from build123d import *

# Parameters (mm, degrees)
SKETCH_1_W          = 54.45
SKETCH_1_H          = 10.46
SKETCH_1_H_2        = 107.75
EXTRUDE_1_DEPTH     = 24.02
CUT_EXTRUDE_1_DEPTH = 10
EXTRUDE_2_DEPTH     = 4.21
SKETCH_4_W          = 3.45
SKETCH_4_H          = 10.08
CUT_EXTRUDE_2_DEPTH = 2
SKETCH_5_W          = 6.71
SKETCH_5_H          = 4.88
CUT_EXTRUDE_4_DEPTH = 134.379468529
SKETCH_7_W          = 5.3
SKETCH_7_H          = 23.4
CUT_EXTRUDE_5_DEPTH = 0.2
SKETCH_8_W          = 10.6
SKETCH_8_H          = 9.42
CUT_EXTRUDE_6_DEPTH = 0.2
SKETCH_9_W          = 10.6
SKETCH_9_H          = 8
CUT_EXTRUDE_7_DEPTH = 0.2
SKETCH_10_W         = 6.68
SKETCH_10_H         = 5.61
CUT_EXTRUDE_8_DEPTH = 2.08


with BuildPart() as part:
    # 草图1 → 凸台-拉伸1 (new body)
    with BuildSketch(Plane(origin=(0, 0, 0), x_dir=(0, 0, -1), z_dir=(1, 0, 0))):
        with Locations((0, 53.875)):
            Rectangle(SKETCH_1_W, SKETCH_1_H)
        with Locations((0, -5.23)):
            Rectangle(SKETCH_1_W, SKETCH_1_H_2)
        Polygon((-37.585, -66.595), (27.225, -59.105), (-27.225, -59.105), (-27.225, 48.645), (-37.585, 48.645), align=None)
        Polygon((-27.225, 59.105), (-37.585, 48.645), (-27.225, 48.645), align=None)
    extrude(amount=EXTRUDE_1_DEPTH)

    # 草图2 → 切除-拉伸1 (cut)
    with BuildSketch(Plane(origin=(0, 59.105, 0), x_dir=(1, 0, 0), z_dir=(0, 1, 0))):
        with BuildLine():
            ThreePointArc((16.585, 17.36), (15.245013524, 20.595013524), (12.01, 21.935))
            Line((12.01, 21.935), (12.01, 12.785))
            ThreePointArc((12.01, 12.785), (15.245013524, 14.124986476), (16.585, 17.36))
        make_face()
        with BuildLine():
            Line((12.01, 12.785), (12.01, 21.935))
            ThreePointArc((12.01, 21.935), (7.435, 17.36), (12.01, 12.785))
        make_face()
    extrude(amount=-CUT_EXTRUDE_1_DEPTH, mode=Mode.SUBTRACT)

    # 草图3 → 凸台-拉伸2 (add)
    with BuildSketch(Plane(origin=(0, 59.105, 0), x_dir=(1, 0, 0), z_dir=(0, 1, 0))):
        with BuildLine():
            ThreePointArc((14.035, 7.04), (13.441891232, 8.471891232), (12.01, 9.065))
            Line((12.01, 9.065), (12.01, 5.015))
            ThreePointArc((12.01, 5.015), (13.441891232, 5.608108768), (14.035, 7.04))
        make_face()
        with BuildLine():
            Line((12.01, 5.015), (12.01, 9.065))
            ThreePointArc((12.01, 9.065), (9.985, 7.04), (12.01, 5.015))
        make_face()
    extrude(amount=EXTRUDE_2_DEPTH)

    # 草图4 → 切除-拉伸2 (cut)
    with BuildSketch(Plane(origin=(0, 59.105, 0), x_dir=(1, 0, 0), z_dir=(0, 1, 0))):
        with Locations((13.735, -6.815)):
            Rectangle(SKETCH_4_W, SKETCH_4_H)
        with Locations((10.285, -6.815)):
            Rectangle(SKETCH_4_W, SKETCH_4_H)
        with Locations((10.285, -20.895)):
            Rectangle(SKETCH_4_W, SKETCH_4_H)
        with Locations((13.735, -20.895)):
            Rectangle(SKETCH_4_W, SKETCH_4_H)
    extrude(amount=-CUT_EXTRUDE_2_DEPTH, mode=Mode.SUBTRACT)

    # 草图5 → 切除-拉伸4 (cut, through all)
    with BuildSketch(Plane(origin=(0, 59.105, 0), x_dir=(1, 0, 0), z_dir=(0, 1, 0))):
        with Locations((3.355, -35.145)):
            Rectangle(SKETCH_5_W, SKETCH_5_H)
        with Locations((20.665, -35.145)):
            Rectangle(SKETCH_5_W, SKETCH_5_H)
    extrude(amount=-CUT_EXTRUDE_4_DEPTH, mode=Mode.SUBTRACT)

    # 草图7 → 切除-拉伸5 (cut)
    with BuildSketch(Plane.XY.offset(37.585)):
        with Locations((9.36, 27.515)):
            Rectangle(SKETCH_7_W, SKETCH_7_H)
        with Locations((14.66, 27.515)):
            Rectangle(SKETCH_7_W, SKETCH_7_H)
    extrude(amount=-CUT_EXTRUDE_5_DEPTH, mode=Mode.SUBTRACT)

    # 草图8 → 切除-拉伸6 (cut)
    with BuildSketch(Plane.XY.offset(37.585)):
        with Locations((12.01, 43.925)):
            Rectangle(SKETCH_8_W, SKETCH_8_H)
    extrude(amount=-CUT_EXTRUDE_6_DEPTH, mode=Mode.SUBTRACT)

    # 草图9 → 切除-拉伸7 (cut)
    with BuildSketch(Plane.XY.offset(37.585)):
        with Locations((12.01, 11.815)):
            Rectangle(SKETCH_9_W, SKETCH_9_H)
    extrude(amount=-CUT_EXTRUDE_7_DEPTH, mode=Mode.SUBTRACT)

    # 草图10 → 切除-拉伸8 (cut)
    with BuildSketch(Plane.ZY):
        with Locations((18.195, 45.12)):
            Rectangle(SKETCH_10_W, SKETCH_10_H)
    extrude(amount=-CUT_EXTRUDE_8_DEPTH, mode=Mode.SUBTRACT)


solid = part.part
Work out the finished part from the listing and answer in its coordinate system (mm). A direction names the side the tool comes from. Round coordinates to 2 decimals unless told otherwise and drop trailing zeros. Write each loop counter-clockwise with the first axis right and the second up, starting at its lowest first coordinate (ties: lowest second). Pieces come first, ordered by that corner, then holes.
1) The mould has two halves that part along Y. Classify faces 5 (the flat face through (11.8, -62.9, 5.6)), 6 (the flat face through (12, 63.315, -7)), 7 (the flat face through (2.08, 45, 18)), 8 (the flat face through (3, -5, 32.705)): pulls with the +Y half, pulls with the -Y half, needs draft (parallel to the pull), parting line crosses it, or undercut.
2) A tool of negligible diameter and unlimited length cuts with its end or side. For faces 1 (the flat face through (21, -5, 32.705)), 2 (the flat face through (12, 29, 37.385)), 3 (the flat face through (12, 57.105, 21)), 4 (the flat face through (6.71, -6, 35)), from which of +Z, -Z, +X, -X, +Y, -Y can it reach the whole face along a straight path? Write none if from no direction.
3) Given pin 1 Ø1 at (x, y) = (0.5, 45.5) entering from +Z (3 decimals); pin 2 Ø5.5 at (x, y) = (14.5, 36) entering from +Z (3 decimals); pin 3 Ø1.7 at (x, z) = (1, 17) entering from -Y, each flat-ended and moving along its own axis, determine where each tip first touches the part or whether it passes through.
4) A cutting plane is placed at B-B (z = -20.5). Give the vertices of the cut face in (x, y) (3 decimals), plus the area to 3 significant figures.
5) A cutting plane is placed at A-A (y = -1). Give the vertices of the cut face in (x, z) (3 decimals), plus the area to 3 significant figures.
6) Straight lines are drawn through the part: line 1 (Z direction, x = 2, y = -44) (3 decimals); line 2 (Z direction, x = 7.25, y = 30) (3 decimals); line 3 (Y direction, x = 5.75, z = 12.5) (3 decimals). For each, find the intervals that lie inside material, in ascending order.
Completed:
1. face 5: pulls with the -Y half
1. face 6: pulls with the +Y half
1. face 7: undercut
1. face 8: needs draft
2. face 1: +Z, +X, +Y, -Y
2. face 2: +Z, +X, -X
2. face 3: +Y
2. face 4: +Z, -X, +Y, -Y
3. pin 1: stops at z = 32.705
3. pin 2: stops at z = 37.385
3. pin 3: stops at y = -64.31
4. outline: (0, -59.882) - (24.02, -59.882) - (24.02, 59.105) - (15.337, 59.105) - (15.337, 49.105) - (8.683, 49.105) - (8.683, 59.105) - (0, 59.105) - close
4. area: 2,790 mm2
5. outline: (0, -27.225) - (24.02, -27.225) - (24.02, 32.705) - (17.31, 32.705) - (17.31, 37.585) - (6.71, 37.585) - (6.71, 32.705) - (0, 32.705) - close
5. area: 1,490 mm2
6. line 1: z = -27.225 to 32.705
6. line 2: z = -27.225 to 37.385
6. line 3: y = -63.696 to 59.105
